Input: part model. Units: mm. Frame: model coordinates. A direction names the side the tool comes from. Round coordinates to 2 decimals unless told otherwise and drop trailing zeros. Write each loop counter-clockwise with the first axis right and the second up, starting at its lowest first coordinate (ties: lowest second). Pieces come first, ordered by that corner, then holes. Notation, with made-up numbers: M 38.25,81.5 L 46.25,81.5 A27 ccw 46.25,117.5 Z; hole C 88.25,-13 d9. An arc over 180 degrees is marked long. Answer as CSV lines item,"result". Start each with the question number.
```python
from build123d import *

# Parameters (mm, degrees)
SKETCH1_W             = 25.4
SKETCH1_H             = 25.4
SKETCH1_W_2           = 22.225
SKETCH1_H_2           = 22.225
BOSS_EXTRUDE1_DEPTH   = 279.4
SKETCH3_W             = 2.4892
SKETCH3_H             = 25.4
SKETCH3_AT_POINT_2_W  = 2.4892
SKETCH3_AT_POINT_2_H  = 25.4
LPATTERN1_START       = -12.7
LPATTERN1_OUTLINE_R   = 2.4892
LPATTERN1_DEPTH       = 25.4
LPATTERN1_2_OUTLINE_R = 2.4892
LPATTERN1_2_DEPTH     = 25.4


# Read off the part's stored shape, not the designer's step: LPattern1
with BuildPart() as part:
    # Sketch1 → Boss-Extrude1 (new, symmetric)
    with BuildSketch(Plane(origin=(0, 0, 0), x_dir=(0, 0, -1), z_dir=(1, 0, 0))):
        Rectangle(SKETCH1_W, SKETCH1_H)
        Rectangle(SKETCH1_W_2, SKETCH1_H_2, mode=Mode.SUBTRACT)
    extrude(amount=BOSS_EXTRUDE1_DEPTH, both=True)

    # Sketch3 → #9 (0.196) Diameter Hole1 (revolve, cut)
    with BuildSketch(Plane(origin=(266.7, 12.7, 0), x_dir=(0, 0, 1), z_dir=(1, 0, 0))):
        with Locations((1.2446, 12.7)):
            Rectangle(SKETCH3_W, SKETCH3_H)
    revolve(axis=Axis((266.7, 19.05, 0), (0, -1, 0)), mode=Mode.SUBTRACT)

    # Sketch3 at point 2 (carried to point 2, square into its face) → #9 (0.196) Diameter Hole1 at 2 (revolve, cut)
    with BuildSketch(Plane(origin=(266.7, 0, 12.7), x_dir=(0, -1, 0), z_dir=(1, 0, 0))):
        with Locations((1.2446, 12.7)):
            Rectangle(SKETCH3_AT_POINT_2_W, SKETCH3_AT_POINT_2_H)
    revolve(axis=Axis((266.7, 0, 19.05), (0, 0, -1)), mode=Mode.SUBTRACT)

    # LPattern1 outline → LPattern1 (cut)
    with BuildSketch(Plane.XY.offset(LPATTERN1_START)):
        with Locations((241.3, 0)):
            Circle(LPATTERN1_OUTLINE_R)
        with Locations((215.9, 0)):
            Circle(LPATTERN1_OUTLINE_R)
        with Locations((190.5, 0)):
            Circle(LPATTERN1_OUTLINE_R)
        with Locations((165.1, 0)):
            Circle(LPATTERN1_OUTLINE_R)
        with Locations((139.7, 0)):
            Circle(LPATTERN1_OUTLINE_R)
        with Locations((114.3, 0)):
            Circle(LPATTERN1_OUTLINE_R)
        with Locations((88.9, 0)):
            Circle(LPATTERN1_OUTLINE_R)
        with Locations((63.5, 0)):
            Circle(LPATTERN1_OUTLINE_R)
        with Locations((38.1, 0)):
            Circle(LPATTERN1_OUTLINE_R)
        with Locations((12.7, 0)):
            Circle(LPATTERN1_OUTLINE_R)
        with Locations((-12.7, 0)):
            Circle(LPATTERN1_OUTLINE_R)
        with Locations((-38.1, 0)):
            Circle(LPATTERN1_OUTLINE_R)
        with Locations((-63.5, 0)):
            Circle(LPATTERN1_OUTLINE_R)
        with Locations((-88.9, 0)):
            Circle(LPATTERN1_OUTLINE_R)
        with Locations((-114.3, 0)):
            Circle(LPATTERN1_OUTLINE_R)
        with Locations((-139.7, 0)):
            Circle(LPATTERN1_OUTLINE_R)
        with Locations((-165.1, 0)):
            Circle(LPATTERN1_OUTLINE_R)
        with Locations((-190.5, 0)):
            Circle(LPATTERN1_OUTLINE_R)
        with Locations((-215.9, 0)):
            Circle(LPATTERN1_OUTLINE_R)
        with Locations((-241.3, 0)):
            Circle(LPATTERN1_OUTLINE_R)
        with Locations((-266.7, 0)):
            Circle(LPATTERN1_OUTLINE_R)
    extrude(amount=LPATTERN1_DEPTH, mode=Mode.SUBTRACT)

    # LPattern1 2 outline → LPattern1 2 (cut)
    with BuildSketch(Plane(origin=(0, 0, 0), x_dir=(1, 0, 0), z_dir=(0, 1, 0)).offset(LPATTERN1_START)):
        with Locations((241.3, 0)):
            Circle(LPATTERN1_2_OUTLINE_R)
        with Locations((215.9, 0)):
            Circle(LPATTERN1_2_OUTLINE_R)
        with Locations((190.5, 0)):
            Circle(LPATTERN1_2_OUTLINE_R)
        with Locations((165.1, 0)):
            Circle(LPATTERN1_2_OUTLINE_R)
        with Locations((139.7, 0)):
            Circle(LPATTERN1_2_OUTLINE_R)
        with Locations((114.3, 0)):
            Circle(LPATTERN1_2_OUTLINE_R)
        with Locations((88.9, 0)):
            Circle(LPATTERN1_2_OUTLINE_R)
        with Locations((63.5, 0)):
            Circle(LPATTERN1_2_OUTLINE_R)
        with Locations((38.1, 0)):
            Circle(LPATTERN1_2_OUTLINE_R)
        with Locations((12.7, 0)):
            Circle(LPATTERN1_2_OUTLINE_R)
        with Locations((-12.7, 0)):
            Circle(LPATTERN1_2_OUTLINE_R)
        with Locations((-38.1, 0)):
            Circle(LPATTERN1_2_OUTLINE_R)
        with Locations((-63.5, 0)):
            Circle(LPATTERN1_2_OUTLINE_R)
        with Locations((-88.9, 0)):
            Circle(LPATTERN1_2_OUTLINE_R)
        with Locations((-114.3, 0)):
            Circle(LPATTERN1_2_OUTLINE_R)
        with Locations((-139.7, 0)):
            Circle(LPATTERN1_2_OUTLINE_R)
        with Locations((-165.1, 0)):
            Circle(LPATTERN1_2_OUTLINE_R)
        with Locations((-190.5, 0)):
            Circle(LPATTERN1_2_OUTLINE_R)
        with Locations((-215.9, 0)):
            Circle(LPATTERN1_2_OUTLINE_R)
        with Locations((-241.3, 0)):
            Circle(LPATTERN1_2_OUTLINE_R)
        with Locations((-266.7, 0)):
            Circle(LPATTERN1_2_OUTLINE_R)
    extrude(amount=LPATTERN1_2_DEPTH, mode=Mode.SUBTRACT)


solid = part.part
```
Item 1: Line query: line 1 (Z direction, x = 54.5, y = -10.5); line 2 (Y direction, x = -266.7, z = -12.2). Output: solid intervals per line, ascending. Write a range as [from, to].
Item 2: Access query for faces 1 (the face through (4, 0, 12.7)), 2 (the face through (4, 0, 11.112)). Directions: +Z, -Z, +X, -X, +Y, -Y. A direction counts if a zero-diameter tool reaches every point of the face in a straight line with its end or side. Return the directions, or none.
Item 3: Draft query along Z for faces 3 (the face through (279.4, 0.1, 11.3)), 4 (the face through (4, 0, -12.7)), 5 (the face through (4, 11.112, 0)). Return one class per face: +Z half, -Z half, draft (parallel to the pull), parting line (faces both ways), or undercut.
Item 4: Cut plane A-A, the plane x = 25.5. Return loops of the section in (y, z).
Results list:
1,line 1,"[-12.7, -11.11], [11.11, 12.7]"
1,line 2,"[-12.7, -2.49], [2.49, 12.7]"
2,face 1,"+Z, +X, -X, +Y, -Y"
2,face 2,"+X, -X"
3,face 3,"draft"
3,face 4,"-Z half"
3,face 5,"undercut"
4,outline,"M -12.7,-12.7 L 12.7,-12.7 L 12.7,12.7 L -12.7,12.7 Z; hole M -11.11,-11.11 L 11.11,-11.11 L 11.11,11.11 L -11.11,11.11 Z"
